Could you check a few things on this model? Use its own coordinates, in mm. Face numbers are marked on the shaded views. A direction names the side the tool comes from. Give positions to 0.01 mm unless a question says otherwise; leave off trailing zeros. Order: outer loops, then holes, each group sorted by start corner. A loop starts at its lowest first (then second) coordinate and runs counter-clockwise, first axis right, second up.
(1) If I drill on probe 1 along X at (y, z) = (7.75, -5.5); probe 2 along Z at (x, y) = (-8.5, 15.5); probe 3 along Z at (x, y) = (0, 16), over which ranges is the centre line in solid material (lowest first)?
(2) Imagine slicing it at B-B, the plane z = 0. Write out the boundary of the cut face in (x, y).
(3) Imagine slicing it at D-D, the plane z = 9. Write out the boundary of the cut face in (x, y).
(4) Will these pins go through, and if not, where does the flat tip stop? pin 1 (1 mm diameter, centred on x = -10.5, y = 16, fed in from +Z); pin 2 (1 mm diameter, centred on y = 11, z = 7, fed in from -X); pin 3 (4 mm diameter, centred on y = 11, z = 6, fed in from +X).
(5) Imagine slicing it at C-C, the plane z = -9.25. Write out the boundary of the cut face in (x, y), then the cut area to 3 significant figures.
(6) If we mould it in two halves opening along Z, with no side actions, what happens to the marked faces 1, 2 and 3? For each: released by +Z, released by -Z, zero draft, split by the parting line, or undercut.
(7) On a 3-axis mill with a long thin cutter (end or side, diameter ignored), from which of +Z, -Z, +X, -X, +Y, -Y can I reach the whole of each face in a straight line? I mean the marked faces 4, 5, 6, 7 and 8. Say none if no direction works.
(8) Imagine slicing it at A-A, the plane x = -9. Write out the boundary of the cut face in (y, z), then the cut area to 3 significant figures.
from build123d import *

# Parameters (mm, degrees)
BOSS_EXTRUDE1_DEPTH      = 12.5
SKETCH2_R                = 1.5
CUT_EXTRUDE1_DEPTH       = 13.5
ESBO_O1_R                = 13.5
ESBO_O1_R_2              = 1.5
ESBO_O1_R_3              = 1.25
RESSALTO_EXTRUS_O1_DEPTH = 6


with BuildPart() as part:
    # Sketch1 → Boss-Extrude1 (new body)
    with BuildSketch(Plane(origin=(0, 0, 0), x_dir=(1, 0, 0), z_dir=(0, 1, 0))):
        with BuildLine():
            ThreePointArc((1.04, 5.400777722), (0.783531714, 6.485041414), (0.31, 7.493590595))
            ThreePointArc((0.31, 7.493590595), (0, 7.5), (-0.31, 7.493590595))
            ThreePointArc((-0.31, 7.493590595), (-0.783531714, 6.485041414), (-1.04, 5.400777722))
            ThreePointArc((-1.04, 5.400777722), (-1.316236154, 5.340179996), (-1.588992288, 5.265463276))
            ThreePointArc((-1.588992288, 5.265463276), (-2.319966139, 6.10634434), (-3.207953823, 6.779309129))
            ThreePointArc((-3.207953823, 6.779309129), (-3.48542379, 6.640920192), (-3.756936559, 6.491180762))
            ThreePointArc((-3.756936559, 6.491180762), (-3.707531894, 5.378093653), (-3.430740821, 4.298839078))
            ThreePointArc((-3.430740821, 4.298839078), (-3.64717462, 4.116809115), (-3.853965592, 3.923894649))
            ThreePointArc((-3.853965592, 3.923894649), (-4.891987708, 4.328757368), (-5.991004086, 4.511969642))
            ThreePointArc((-5.991004086, 4.511969642), (-6.172378994, 4.2604856), (-6.343204228, 4.001719645))
            ThreePointArc((-6.343204228, 4.001719645), (-5.782181198, 3.039089449), (-5.035540265, 2.212088208))
            ThreePointArc((-5.035540265, 2.212088208), (-5.142589335, 1.950326879), (-5.236041824, 1.683409046))
            ThreePointArc((-5.236041824, 1.683409046), (-6.343313848, 1.559504249), (-7.401587511, 1.210992284))
            ThreePointArc((-7.401587511, 1.210992284), (-7.445316556, 0.904025102), (-7.476320253, 0.595512782))
            ThreePointArc((-7.476320253, 0.595512782), (-6.532202472, 0.003866477), (-5.486758119, -0.381425412))
            ThreePointArc((-5.486758119, -0.381425412), (-5.459898808, -0.662951741), (-5.418603976, -0.942725282))
            ThreePointArc((-5.418603976, -0.942725282), (-6.341463231, -1.567012498), (-7.116556437, -2.367408811))
            ThreePointArc((-7.116556437, -2.367408811), (-7.01262182, -2.659536653), (-6.896701407, -2.947118882))
            ThreePointArc((-6.896701407, -2.947118882), (-5.785774881, -3.032242258), (-4.68102581, -2.887559066))
            ThreePointArc((-4.68102581, -2.887559066), (-4.526411262, -3.124356107), (-4.359829258, -3.352892609))
            ThreePointArc((-4.359829258, -3.352892609), (-4.886859811, -4.334545567), (-5.201208047, -5.403465078))
            ThreePointArc((-5.201208047, -5.403465078), (-4.973419937, -5.613830611), (-4.737131383, -5.814601127))
            ThreePointArc((-4.737131383, -5.814601127), (-3.713895991, -5.373700834), (-2.802926901, -4.732187738))
            ThreePointArc((-2.802926901, -4.732187738), (-2.555977446, -4.870008141), (-2.302270198, -4.994952646))
            ThreePointArc((-2.302270198, -4.994952646), (-2.312735701, -6.109086484), (-2.094325574, -7.201652615))
            ThreePointArc((-2.094325574, -7.201652615), (-1.794867482, -7.282063631), (-1.492341648, -7.350028327))
            ThreePointArc((-1.492341648, -7.350028327), (-0.791208287, -6.484109309), (-0.282711218, -5.492729228))
            ThreePointArc((-0.282711218, -5.492729228), (0, -5.5), (0.282711218, -5.492729228))
            ThreePointArc((0.282711218, -5.492729228), (0.791208287, -6.484109309), (1.492341648, -7.350028327))
            ThreePointArc((1.492341648, -7.350028327), (1.794867482, -7.282063631), (2.094325574, -7.201652615))
            ThreePointArc((2.094325574, -7.201652615), (2.312735701, -6.109086484), (2.302270198, -4.994952646))
            ThreePointArc((2.302270198, -4.994952646), (2.555977446, -4.870008141), (2.802926901, -4.732187738))
            ThreePointArc((2.802926901, -4.732187738), (3.713895991, -5.373700834), (4.737131383, -5.814601127))
            ThreePointArc((4.737131383, -5.814601127), (4.973419937, -5.613830611), (5.201208047, -5.403465078))
            ThreePointArc((5.201208047, -5.403465078), (4.886859811, -4.334545567), (4.359829258, -3.352892609))
            ThreePointArc((4.359829258, -3.352892609), (4.526411262, -3.124356107), (4.68102581, -2.887559066))
            ThreePointArc((4.68102581, -2.887559066), (5.785774881, -3.032242258), (6.896701407, -2.947118882))
            ThreePointArc((6.896701407, -2.947118882), (7.01262182, -2.659536653), (7.116556437, -2.367408811))
            ThreePointArc((7.116556437, -2.367408811), (6.341463231, -1.567012498), (5.418603976, -0.942725282))
            ThreePointArc((5.418603976, -0.942725282), (5.459898808, -0.662951741), (5.486758119, -0.381425412))
            ThreePointArc((5.486758119, -0.381425412), (6.532202472, 0.003866477), (7.476320253, 0.595512782))
            ThreePointArc((7.476320253, 0.595512782), (7.445316556, 0.904025102), (7.401587511, 1.210992284))
            ThreePointArc((7.401587511, 1.210992284), (6.343313848, 1.559504249), (5.236041824, 1.683409046))
            ThreePointArc((5.236041824, 1.683409046), (5.142589335, 1.950326879), (5.035540265, 2.212088208))
            ThreePointArc((5.035540265, 2.212088208), (5.782181198, 3.039089449), (6.343204228, 4.001719645))
            ThreePointArc((6.343204228, 4.001719645), (6.172378994, 4.2604856), (5.991004086, 4.511969642))
            ThreePointArc((5.991004086, 4.511969642), (4.891987708, 4.328757368), (3.853965592, 3.923894649))
            ThreePointArc((3.853965592, 3.923894649), (3.64717462, 4.116809115), (3.430740821, 4.298839078))
            ThreePointArc((3.430740821, 4.298839078), (3.707531894, 5.378093653), (3.756936559, 6.491180762))
            ThreePointArc((3.756936559, 6.491180762), (3.48542379, 6.640920192), (3.207953823, 6.779309129))
            ThreePointArc((3.207953823, 6.779309129), (2.319966139, 6.10634434), (1.588992288, 5.265463276))
            ThreePointArc((1.588992288, 5.265463276), (1.316236154, 5.340179996), (1.04, 5.400777722))
        make_face()
    extrude(amount=BOSS_EXTRUDE1_DEPTH)

    # Sketch2 → Cut-Extrude1 (cut, through all)
    with BuildSketch(Plane(origin=(0, 12.5, 0), x_dir=(1, 0, 0), z_dir=(0, 1, 0))):
        Circle(SKETCH2_R)
    extrude(amount=-CUT_EXTRUDE1_DEPTH, mode=Mode.SUBTRACT)

    # Esboço1 → Ressalto-extrusão1 (add)
    with BuildSketch(Plane(origin=(0, 12.5, 0), x_dir=(1, 0, 0), z_dir=(0, 1, 0))):
        Circle(ESBO_O1_R)
        Circle(ESBO_O1_R_2, mode=Mode.SUBTRACT)
        with Locations((9.22317055, 5.325)):
            Circle(ESBO_O1_R_3, mode=Mode.SUBTRACT)
        with Locations((9.22317055, -5.325)):
            Circle(ESBO_O1_R_3, mode=Mode.SUBTRACT)
        with Locations((-9.22317055, -5.325)):
            Circle(ESBO_O1_R_3, mode=Mode.SUBTRACT)
        with Locations((-9.22317055, 5.325)):
            Circle(ESBO_O1_R_3, mode=Mode.SUBTRACT)
    extrude(amount=RESSALTO_EXTRUS_O1_DEPTH)


solid = part.part
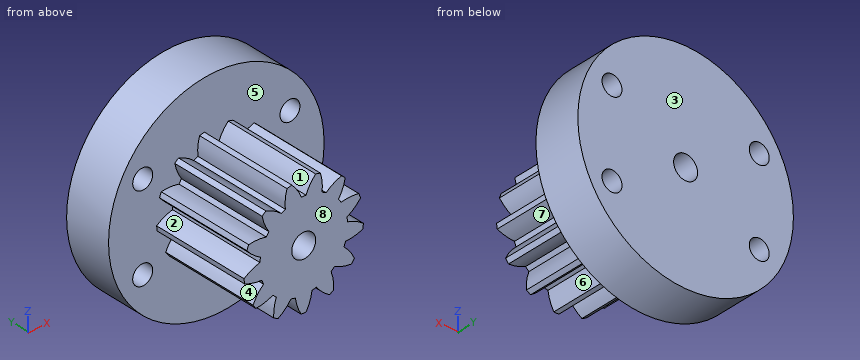
Answer block:
1. probe 1: x = -3.72 to -1.76, -1.03 to 1.03, 1.76 to 3.72
1. probe 2: z = -10.49 to -6.34, -4.31 to 4.31, 6.34 to 10.49
1. probe 3: z = -13.5 to -1.5, 1.5 to 13.5
2. outline: (-13.5, 12.5) - (-6.52, 12.5) - (-6.52, 0) - (-1.5, 0) - (-1.5, 18.5) - (-13.5, 18.5) - close; (1.5, 0) - (6.52, 0) - (6.52, 12.5) - (13.5, 12.5) - (13.5, 18.5) - (1.5, 18.5) - close
3. outline: (-10.06, 12.5) - (10.06, 12.5) - (10.06, 18.5) - (-10.06, 18.5) - close
4. pin 1: stops at z = 9.07
4. pin 2: stops at x = -2.26
4. pin 3: stops at x = 12.66
5. outline: (-9.83, 12.5) - (9.83, 12.5) - (9.83, 18.5) - (-9.83, 18.5) - close
5. area: 118 mm2
6. face 1: released by +Z
6. face 2: undercut
6. face 3: zero draft
7. face 4: -X, -Y
7. face 5: -Y
7. face 6: -Z, -Y
7. face 7: +X, -Y
7. face 8: +Z, -Z, +X, -X, -Y
8. outline: (12.5, -10.06) - (18.5, -10.06) - (18.5, -6.55) - (12.5, -6.55) - close; (12.5, -4.1) - (18.5, -4.1) - (18.5, 4.1) - (12.5, 4.1) - close; (12.5, 6.55) - (18.5, 6.55) - (18.5, 10.06) - (12.5, 10.06) - close
8. area: 91.2 mm2
